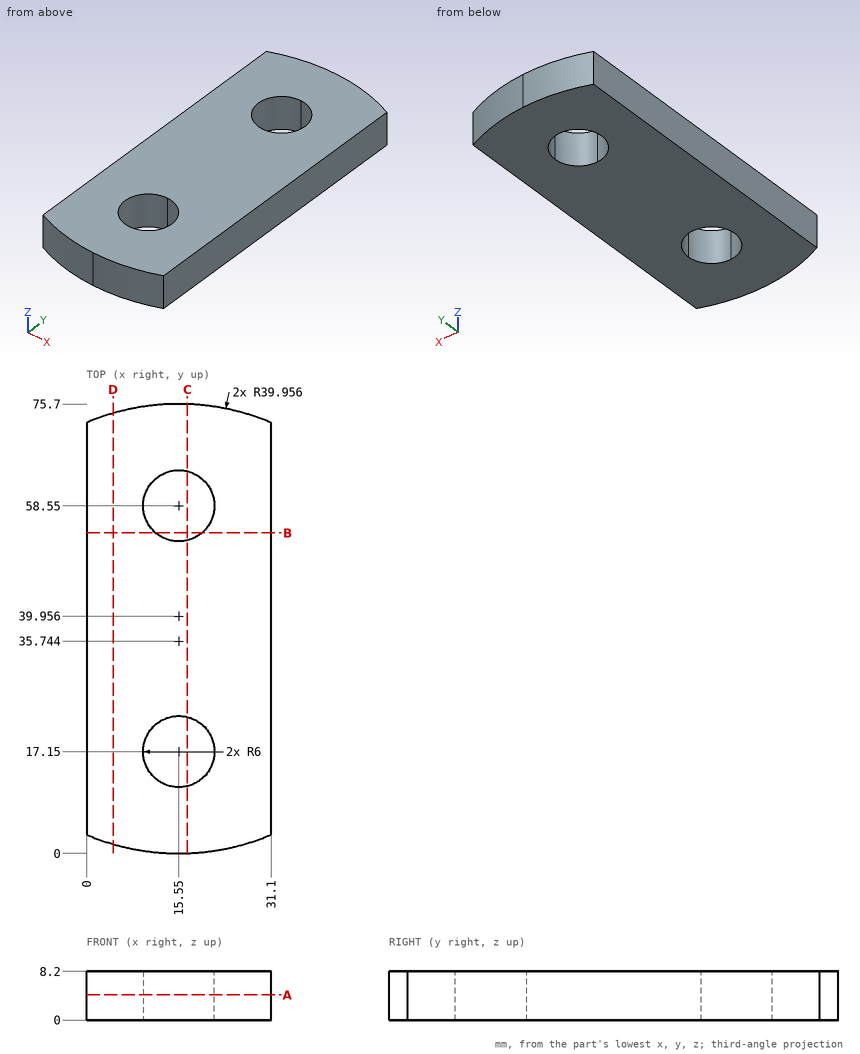
The figure shows three views and two pictorial views of one solid part (mm, origin at its lowest corner). Answer the questions. Coordinates: 2 decimals unless noted, no trailing zeros. Loops run counter-clockwise (first coordinate to the right, second up) from the corner with the lowest first, then second, coordinate; pieces in that order, holes last.
1) Find section C-C on x = 17. Write down the section's boundary in (y, z), then the cut area to 3 significant figures.
2) Find section B-B on y = 54. Write down the section's boundary in (x, z), then the cut area to 3 significant figures.
3) Find section D-D on x = 4.5. Write down the section's boundary in (y, z), then the cut area to 3 significant figures.
4) Flat-ended cylindrical pins translate along their axes: pin 1 Ø1.5 at (x, z) = (3.5, 3) entering from +Y; pin 2 Ø4 at (x, z) = (26.5, 4) entering from -Y (1 decimal); pin 3 Ø1 at (x, z) = (9, 7.5) entering from -Y. Find the tip coordinate at first contact, or state that the pin passes through.
5) Find section A-A on z = 4.25. Write down the section's boundary in (x, y).
6) Find the intervals of material crossed by L1, parallel to Y at x = 15.5, z = 2.25; L2, parallel to Y at x = 18.5, z = 5 (1 decimal); L3, parallel to X at y = 55, z = 3, in increasing order.
Values:
1. outline: (0.03, 0) - (11.33, 0) - (11.33, 8.2) - (0.03, 8.2) - close; (22.97, 0) - (52.73, 0) - (52.73, 8.2) - (22.97, 8.2) - close; (64.37, 0) - (75.67, 0) - (75.67, 8.2) - (64.37, 8.2) - close
1. area: 429 mm2
2. outline: (0, 0) - (11.64, 0) - (11.64, 8.2) - (0, 8.2) - close; (19.46, 0) - (31.1, 0) - (31.1, 8.2) - (19.46, 8.2) - close
2. area: 191 mm2
3. outline: (1.56, 0) - (74.14, 0) - (74.14, 8.2) - (1.56, 8.2) - close
3. area: 595 mm2
4. pin 1: stops at y = 74.07
4. pin 2: stops at y = 1
4. pin 3: stops at y = 0.46
5. outline: (0, 3.15) arc R39.96 ccw to (31.1, 3.15) - (31.1, 72.55) arc R39.96 ccw to (0, 72.55) - close; hole circle Ø12 at (15.55, 17.15); hole circle Ø12 at (15.55, 58.55)
6. L1: y = 0 to 11.15, 23.15 to 52.55, 64.55 to 75.7
6. L2: y = 0.1 to 11.9, 22.4 to 53.3, 63.8 to 75.6
6. L3: x = 0 to 10.71, 20.39 to 31.1
